Job drawing, mm, ordinate dimensions from the low corner. One solid piece. Give positions to 0.01 mm unless a question says otherwise; leave off trailing zeros. Order: outer loops, then holes, each group sorted by start corner. A loop starts at its lowest first (then second) coordinate and runs counter-clockwise, first axis right, second up. Notation, with made-up numbers: (39, -31.5) - (87, -31.5) arc R36 ccw to (87, 6.5) - close; hole circle Ø8 at (38.25, -28.5). An arc over 180 degrees is marked (long way). One line per item, written item: value.
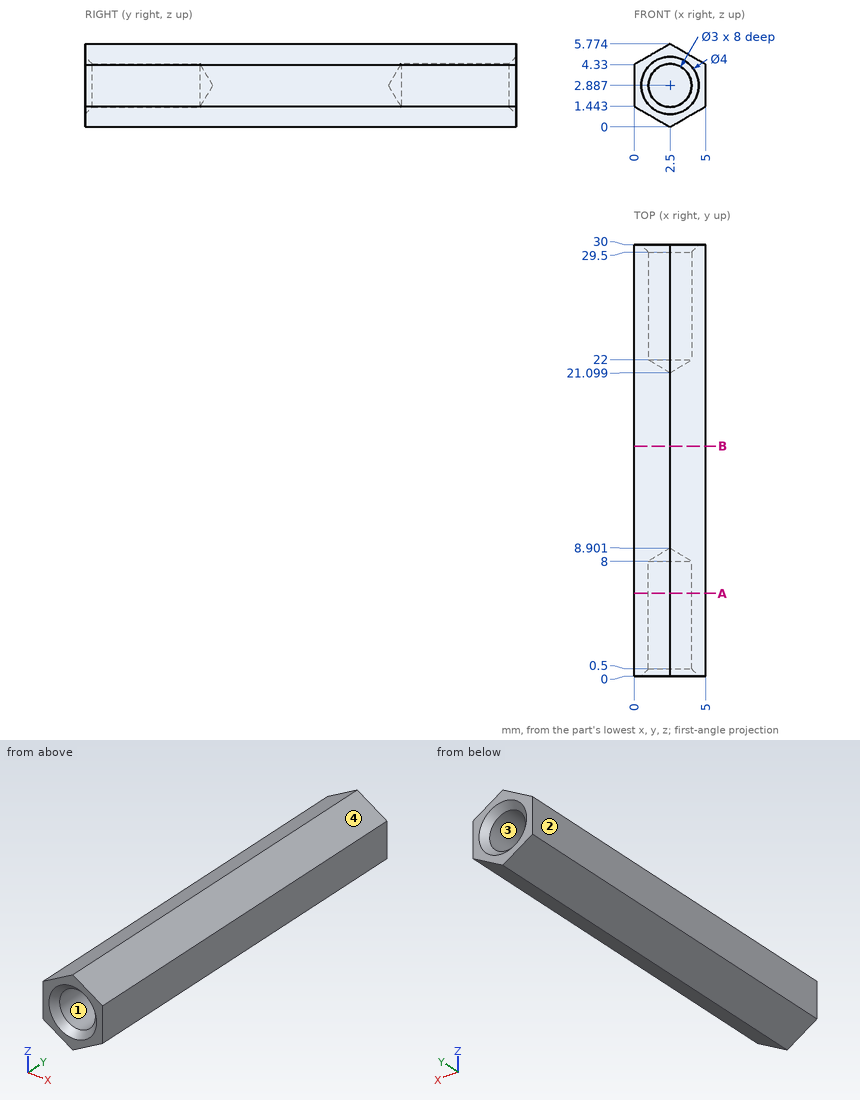
1) Slice it at A-A on y = 5.75. Write the cut outline in (x, z).
Answer:
outline: (0, 1.44) - (2.5, 0) - (5, 1.44) - (5, 4.33) - (2.5, 5.77) - (0, 4.33) - close; hole circle Ø3 at (2.5, 2.89)
2) Slice it at B-B on y = 16. Write the cut outline in (x, z).
Answer:
outline: (0, 1.44) - (2.5, 0) - (5, 1.44) - (5, 4.33) - (2.5, 5.77) - (0, 4.33) - close
3) Wall check: line 1 along X through (y, z) = (6, 3.8); line 2 along Z through (x, y) = (3.5, 28.75) (1 decimal); line 3 along Z through (x, y) = (2.75, 22.5) (1 decimal). Give the ranges that are in metal, low to high. Write a range as [from, to].
Answer:
line 1: x = [0, 1.31], [3.69, 5]
line 2: z = [0.6, 1.8], [4, 5.2]
line 3: z = [0.1, 1.4], [4.4, 5.6]
4) Two-plate mould, pull along X, no slides. Class the marked faces 1, 2, 3 and 4: pulls with the +X half, pulls with the -X half, needs draft (parallel to the pull), parting line crosses it, or undercut.
Answer:
face 1: undercut
face 2: pulls with the -X half
face 3: undercut
face 4: pulls with the +X half
5) Drop flat-ended pins along their axis: P1, Ø1, axis at x = 1.5, y = 13, coming from the +Z side (1 decimal); P2, Ø1.5, axis at x = 2, y = 5.5, coming from the -Z side; P3, Ø2.5, axis at x = 2.5, z = 2.89, coming from the +Y side. Give the stop position or say it passes through.
Answer:
P1: stops at z = 5.5
P2: stops at z = 0
P3: stops at y = 21.85
